Solid Edge part; units mm, degrees
sketch "Sketch1" plane through (0, 0, 0) normal (0, 0, 1) x (1, 0, 0)
  circle A0 centre (0, 0) radius 4
extrude "Protrusion1" add sketch "Sketch1" along normal blind 7
sketch "Sketch2" plane through (0, 0, 0) normal (0, 0, -1) x (-1, 0, 0)
  line L0 (-4, 4) -> (4, 4)
  line L1 (4, 4) -> (4, -4)
  line L2 (4, -4) -> (-4, -4)
  line L3 (-4, -4) -> (-4, 4)
extrude "ExtrudedProtrusion_2" add sketch "Sketch2" along normal blind 13.5
sketch "Sketch3" plane through (0, 0, -13.5) normal (0, 0, -1) x (-1, 0, 0)
  arc A0 (-4, 4) -> (-12, -4) centre (-4, -4) ccw
  line L0 (-12, -4) -> (-12, -24)
  line L1 (-12, -24) -> (-6, -24)
  line L2 (-6, -24) -> (-6, -4)
  line L3 (-6, -4) -> (6, -4)
  line L4 (6, -24) -> (6, -4)
  line L5 (12, -24) -> (6, -24)
  line L6 (12, -4) -> (12, -24)
  arc A1 (4, 4) -> (12, -4) centre (4, -4) cw
  line L7 (-4, 4) -> (4, 4)
  dimension "D1" = 12
extrude "Protrusion2" add sketch "Sketch3" against normal up to vertex (13.5 mm away)
sketch "Sketch4" plane through (0, 4, -1.5) normal (0, 1, 0) x (0, 0, -1)
  circle A0 centre (2.5, 0) radius 2.6
extrude "Cutout1" cut sketch "Sketch4" against normal through all
fillet "Round_3" radius 10 2 edges at (-9, -24, 0) (9, -24, 0)
sketch "Sketch5" plane through (0, 0, 7) normal (0, 0, 1) x (0, -1, 0)
  circle A0 centre (0, 0) radius 2.25
extrude "ExtrudedCutout_2" cut sketch "Sketch5" against normal blind 6
Input: part model. Units: mm. Frame: model coordinates. A direction names the side the tool comes from. Coordinates: 2 decimals unless noted, no trailing zeros. Loops run counter-clockwise (first coordinate to the right, second up) from the corner with the lowest first, then second, coordinate; pieces in that order, holes last. Notation, with made-up numbers: M -19,49.5 L 14,49.5 A12 ccw 14,58.5 Z; hole C 40,74.25 d11. An arc over 180 degrees is marked long. One line per item, written item: value.
(1) Pin query (flat end, axial travel): pin 1 (8 mm diameter, centred on x = -2.5, y = -16.5, fed in from +Z); pin 2 (1 mm diameter, centred on y = 1, z = -2.5, fed in from +X); pin 3 (2 mm diameter, centred on y = -13, z = 2, fed in from +X); pin 4 (2.5 mm diameter, centred on x = 0, y = 0, fed in from +Z). Return the tip coordinate at first contact, or that it passes through.
Filled in:
pin 1: z = -0.02
pin 2: x = 10.61
pin 3: through
pin 4: z = 1
(2) Section C-C (z = -4). Output: boundary loops of the cut face in (x, y), and give its area (3 significant figures).
Filled in:
outline: M -12,-22 L -6,-22 L -6,-4 L -2.6,-4 L -2.6,4 L -4,4 A8 ccw -12,-4 Z; M 2.6,-4 L 6,-4 L 6,-22 L 12,-22 L 12,-4 A8 ccw 4,4 L 2.6,4 Z
area: 339 mm^2
(3) Section A-A (y = -10). Output: boundary loops of the cut face in (x, z), and give its area (3 significant figures).
Filled in:
outline: M -12,-13.5 L -6,-13.5 L -6,0 L -12,0 Z; M 6,-13.5 L 12,-13.5 L 12,0 L 6,0 Z
area: 162 mm^2
(4) Line query: line 1 along X through (y, z) = (0, 3.3); line 2 along Z through (x, y) = (0, 1.5); line 3 along X through (y, z) = (-10.75, -3.5). Output: solid intervals per line, ascending. Write a range as from..to.
Filled in:
line 1: -4..-2.25, 2.25..4
line 2: -13.5..-6.6, -1.4..1
line 3: -12..-6, 6..12
(5) Pull-direction query (Z, two-part tool) for faces 1 (the cylindrical face through (-0.1, 0.1, -1.4)), 2 (the cylindrical face through (8.96, -21.15, -3.01)), 3 (the cylindrical face through (2.23, 0.29, 4.04)), 4 (the flat face through (-0.2, -3.6, -13.5)); classes: +Z half, -Z half, draft (parallel to the pull), parting line (faces both ways), or undercut.
Filled in:
face 1: undercut
face 2: +Z half
face 3: draft
face 4: -Z half
(6) Section D-D (y = -22). Output: boundary loops of the cut face in (x, z).
Filled in:
outline: M -12,-13.5 L -6,-13.5 L -6,-4 L -12,-4 Z; M 6,-13.5 L 12,-13.5 L 12,-4 L 6,-4 Z
(7) Reachability of faces 5 (the flat face through (6, -14, -7)), 6 (the flat face through (2, -2, 7)), 7 (the flat face through (0, 0, 1)) from +Z, -Z, +X, -X, +Y, -Y: full face, straight path, thin tool, end or side. Return the list, or none.
Filled in:
face 5: +Z, -Z, -Y
face 6: +Z, +X, -X, +Y, -Y
face 7: +Z
(8) Section B-B (z = -10.5). Output: boundary loops of the cut face in (x, y), and give its area (3 significant figures).
Filled in:
outline: M -12,-24 L -6,-24 L -6,-4 L 6,-4 L 6,-24 L 12,-24 L 12,-4 A8 ccw 4,4 L -4,4 A8 ccw -12,-4 Z
area: 405 mm^2
